```python
from build123d import *

# Parameters (mm, degrees)
SKETCH1_W           = 254
SKETCH1_H           = 254
SKETCH1_W_2         = 3.175
SKETCH1_H_2         = 38.1
SKETCH1_H_3         = 34.925
SKETCH1_W_3         = 38.1
SKETCH1_H_4         = 3.175
SKETCH1_W_4         = 34.925
BOSS_EXTRUDE1_DEPTH = 3.175


with BuildPart() as part:
    # Sketch1 → Boss-Extrude1 (new body)
    with BuildSketch(Plane(origin=(0, 0, 0), x_dir=(1, 0, 0), z_dir=(0, 1, 0))):
        Rectangle(SKETCH1_W, SKETCH1_H)
        Polygon((-111.125, 114.3), (-76.2, 114.3), (-38.1, 114.3), (-12.7, 114.3), (-12.7, 117.602), (12.7, 117.602), (12.7, 114.3), (38.1, 114.3), (76.2, 114.3), (111.125, 114.3), (114.3, 114.3), (114.3, 111.125), (114.3, 76.2), (114.3, 38.1), (114.3, 12.7), (117.602, 12.7), (117.602, -12.7), (114.3, -12.7), (114.3, -38.1), (114.3, -76.2), (114.3, -111.125), (114.3, -114.3), (111.125, -114.3), (76.2, -114.3), (38.1, -114.3), (12.7, -114.3), (12.7, -117.602), (-12.7, -117.602), (-12.7, -114.3), (-38.1, -114.3), (-76.2, -114.3), (-111.125, -114.3), (-114.3, -114.3), (-114.3, -111.125), (-114.3, -76.2), (-114.3, -38.1), (-114.3, -12.7), (-117.602, -12.7), (-117.602, 12.7), (-114.3, 12.7), (-114.3, 38.1), (-114.3, 76.2), (-114.3, 111.125), (-114.3, 114.3), align=None, mode=Mode.SUBTRACT)
        Polygon((-38.1, 111.125), (-76.2, 111.125), (-111.125, 111.125), (-111.125, 76.2), (-111.125, 38.1), (-111.125, 0), (-111.125, -38.1), (-111.125, -76.2), (-111.125, -111.125), (-76.2, -111.125), (-38.1, -111.125), (0, -111.125), (38.1, -111.125), (76.2, -111.125), (111.125, -111.125), (111.125, -76.2), (111.125, -38.1), (111.125, 0), (111.125, 38.1), (111.125, 76.2), (111.125, 111.125), (76.2, 111.125), (38.1, 111.125), (0, 111.125), align=None)
        with Locations((-112.7125, 57.15)):
            Rectangle(SKETCH1_W_2, SKETCH1_H_2)
        Polygon((-111.125, -38.1), (-111.125, 0), (-114.3, 0), (-114.3, -12.7), (-114.3, -38.1), align=None)
        with Locations((-112.7125, -93.6625)):
            Rectangle(SKETCH1_W_2, SKETCH1_H_3)
        with Locations((-57.15, -112.7125)):
            Rectangle(SKETCH1_W_3, SKETCH1_H_4)
        Polygon((38.1, -111.125), (0, -111.125), (0, -114.3), (12.7, -114.3), (38.1, -114.3), align=None)
        with Locations((93.6625, -112.7125)):
            Rectangle(SKETCH1_W_4, SKETCH1_H_4)
        with Locations((112.7125, -57.15)):
            Rectangle(SKETCH1_W_2, SKETCH1_H_2)
        Polygon((114.3, 38.1), (111.125, 38.1), (111.125, 0), (114.3, 0), (114.3, 12.7), align=None)
        with Locations((112.7125, 93.6625)):
            Rectangle(SKETCH1_W_2, SKETCH1_H_3)
        with Locations((57.15, 112.7125)):
            Rectangle(SKETCH1_W_3, SKETCH1_H_4)
        Polygon((-12.7, 114.3), (-38.1, 114.3), (-38.1, 111.125), (0, 111.125), (0, 114.3), align=None)
        with Locations((-93.6625, 112.7125)):
            Rectangle(SKETCH1_W_4, SKETCH1_H_4)
    extrude(amount=BOSS_EXTRUDE1_DEPTH)


solid = part.part
```
Could you check a few things on this model? Use its own coordinates, in mm. Round coordinates to 2 decimals unless told otherwise and drop trailing zeros. Order: outer loops, then holes, each group sorted by start corner. A loop starts at its lowest first (then second) coordinate and runs counter-clockwise, first axis right, second up. Notation, with made-up numbers: M 1.25,-29 L 26.25,-29 A22 ccw 26.25,-9 Z; hole C 86.25,-40 d11. An arc over 180 degrees is marked long. One line per question, with ' | ' between items. Start each with the question number.
(1) For P1, Ø1.5, axis at x = -0.5, z = -52, coming from the -Y side, with a flat end and sliding along its axis, tell me the tip position at first contact or that it passes through.
(2) Please list where these lines run through material, in increasing order: line 1 along X through (y, z) = (2.6, -2) (3 decimals); line 2 along X through (y, z) = (2.4, 6) (3 decimals); line 3 along X through (y, z) = (0.8, -37.5) (3 decimals).
(3) Suppose I cut it at B-B on y = 1.55. Count the separate pieces of the cut face and the enclosed holes in it, then the cut area to 3 significant figures.
(4) Suppose I cut it at A-A on z = -4. List the corners of the cut face in (x, y) for me (3 decimals).
Geometry results:
1) P1: y = 0
2) line 1: -127 to -117.602, -111.125 to 114.3, 117.602 to 127 | line 2: -127 to -117.602, -114.3 to 111.125, 117.602 to 127 | line 3: -127 to -114.3, -111.125 to 127
3) separate pieces: 1 | enclosed holes: 12 | area: 62,700 mm²
4) outline: M -127,0 L -117.602,0 L -117.602,3.175 L -127,3.175 Z; M -111.125,0 L 114.3,0 L 114.3,3.175 L -111.125,3.175 Z; M 117.602,0 L 127,0 L 127,3.175 L 117.602,3.175 Z
